```python
from build123d import *

# Parameters (mm, degrees)
F0_R     = 11.75
F1_DEPTH = 8
F2_T     = -2.5
F3_W     = 3.3
F3_H     = 4
F4_DEPTH = 25


with BuildPart() as f1:
    # F0 (on Right) → F1 (new body)
    with BuildSketch(Plane.YZ):
        with Locations((-7.938508, 23.813721)):
            Circle(F0_R)
    extrude(amount=F1_DEPTH)

    # F2
    f2_openings = [f1.faces().sort_by_distance(p)[0] for p in [
        (8, -7.938508, 23.813721),
    ]]
    offset(amount=F2_T, openings=f2_openings)

    # F3 (on Top) → F4 (cut)
    with BuildSketch(Plane.XY):
        with Locations((4.21131, -7.012647)):
            Rectangle(F3_W, F3_H)
    extrude(amount=F4_DEPTH, mode=Mode.SUBTRACT)


solid = f1.part
```
Design review of the part built by this model. Coordinates are the model's own, in mm. A direction names the side the tool comes from. Give positions to 0.01 mm unless a question says otherwise; leave off trailing zeros. Write each loop counter-clockwise with the first axis right and the second up, starting at its lowest first coordinate (ties: lowest second). Pieces come first, ordered by that corner, then holes. Notation, with made-up numbers: (59.5, -15.5) - (89.5, -15.5) arc R30 cw to (89.5, 13.5) - close; hole circle Ø8 at (-33.75, 23). An arc over 180 degrees is marked (long way). Return JSON: item names as keys, results as strings. Group by question number.
(1) Machinability: for faces 4 (the flat face through (8, -8, 14)), 5 (the flat face through (5.861, -7, 14)), 6 (the cylindrical face through (5.212, -9.143, 32.985)), which of the approach directions +Z, -Z, +X, -X, +Y, -Y give a long, thin tool a straight path to every point of the face, cutting with its end or side? Answer none if there is none.
(2) We need section C-C, the plane x = 6.25. Give the boundary of the cut face in (y, z).
(3) We need section D-D, the plane x = 1. Give the boundary of the cut face in (y, z).
(4) We need section B-B, the plane z = 22.5. Give the boundary of the cut face in (x, y).
(5) To check wall thickness, follow probe 1 along X at (y, z) = (-8.25, 14); probe 2 along Z at (x, y) = (1.5, -7.75); probe 3 along Y at (x, z) = (3.75, 14.25). State the ranges of each line that lie inside material, in increasing order.
(6) We need section A-A, the plane y = -16. Give the boundary of the cut face in (x, z), then the cut area to 3 significant figures.
(7) Insertion check: pin 1 (1 mm diameter, centred on x = 4, y = -9, fed in from +Z); pin 2 (2 mm diameter, centred on x = 4.5, y = -9.5, fed in from -Z); pin 3 (1 mm diameter, centred on x = 3, y = -4, fed in from +Z). Each pin has a flat end and moves straight along its axis. Give the tip position at first contact, or say it passes through.
(8) Mouldability with a two-part tool opening along Y and no side actions: class faces 1 (the cylindrical face through (3.944, 2.916, 19.313)), 2 (the flat face through (4, -5.013, 14)), 3 (the flat face through (0, -8, 24)) as +Y half, -Y half, draft (parallel to the pull), parting line (faces both ways), or undercut.
Reported:
{
 "1": {"face 4": "+Z, -Z, +X, +Y, -Y", "face 5": "-Z", "face 6": "+X"},
 "2": {"outline": "circle Ø23.5 at (-7.94, 23.81); hole circle Ø18.5 at (-7.94, 23.81)"},
 "3": {"outline": "circle Ø23.5 at (-7.94, 23.81)"},
 "4": {"outline": "(0, -19.61) - (8, -19.61) - (8, -17.09) - (2.5, -17.09) - (2.5, 1.22) - (8, 1.22) - (8, 3.74) - (0, 3.74) - close"},
 "5": {"probe 1": "x = 0 to 2.56, 5.86 to 8", "probe 2": "z = 12.07 to 35.56", "probe 3": "y = -14.76 to -9.01, -5.01 to -1.11"},
 "6": {"outline": "(0, 15.27) - (8, 15.27) - (8, 19.28) - (2.5, 19.28) - (2.5, 28.35) - (8, 28.35) - (8, 32.36) - (0, 32.36) - close", "area": "86.9 mm2"},
 "7": {"pin 1": "stops at z = 35.55", "pin 2": "stops at z = 12.11", "pin 3": "stops at z = 35.05"},
 "8": {"face 1": "parting line", "face 2": "undercut", "face 3": "draft"}
}
